from build123d import *

# Parameters (mm, degrees)
SKETCH1_W           = 250
SKETCH1_H           = 250
SKETCH1_R           = 1.5
BOSS_EXTRUDE1_DEPTH = 1.5
SKETCH2_R           = 2.25
SKETCH2_R_2         = 1.5
CUT_EXTRUDE1_DEPTH  = 2
CUT_EXTRUDE2_DEPTH  = 2
CUT_EXTRUDE3_DEPTH  = 2


with BuildPart() as part:
    # Sketch1 → Boss-Extrude1 (new body)
    with BuildSketch(Plane(origin=(0, 0, 0), x_dir=(1, 0, 0), z_dir=(0, 1, 0))):
        with Locations((-125, -125)):
            Rectangle(SKETCH1_W, SKETCH1_H)
        with Locations(Location((-125, -5.475, 0), (0, 0, 270))):
            Circle(SKETCH1_R, mode=Mode.SUBTRACT)
        with Locations(Location((-11.32496989, -88.064743747, 0), (0, 0, 270))):
            Circle(SKETCH1_R, mode=Mode.SUBTRACT)
        with Locations(Location((-54.74496772, -28.302243747, 0), (0, 0, 270))):
            Circle(SKETCH1_R, mode=Mode.SUBTRACT)
        with Locations(Location((-11.32496989, -161.935256253, 0), (0, 0, 270))):
            Circle(SKETCH1_R, mode=Mode.SUBTRACT)
        with Locations(Location((-54.74496772, -221.697756253, 0), (0, 0, 269.999999999))):
            Circle(SKETCH1_R, mode=Mode.SUBTRACT)
        with Locations(Location((-125, -244.525, 0), (0, 0, 270))):
            Circle(SKETCH1_R, mode=Mode.SUBTRACT)
        with Locations(Location((-195.25503228, -221.697756253, 0), (0, 0, 269.999999999))):
            Circle(SKETCH1_R, mode=Mode.SUBTRACT)
        with Locations(Location((-238.67503011, -161.935256253, 0), (0, 0, 270))):
            Circle(SKETCH1_R, mode=Mode.SUBTRACT)
        with Locations(Location((-238.67503011, -88.064743747, 0), (0, 0, 270))):
            Circle(SKETCH1_R, mode=Mode.SUBTRACT)
        with Locations(Location((-195.25503228, -28.302243747, 0), (0, 0, 270))):
            Circle(SKETCH1_R, mode=Mode.SUBTRACT)
    extrude(amount=BOSS_EXTRUDE1_DEPTH)

    # Sketch2 → Cut-Extrude1 (cut)
    with BuildSketch(Plane(origin=(0, 1.5, 0), x_dir=(1, 0, 0), z_dir=(0, 1, 0))):
        with Locations(Location((-212.5, -125, 0), (0, 0, 270))):
            Circle(SKETCH2_R)
        with Locations(Location((-228, -140.5, 0), (0, 0, 270))):
            Circle(SKETCH2_R_2)
        with Locations(Location((-228, -109.5, 0), (0, 0, 270))):
            Circle(SKETCH2_R_2)
        with Locations(Location((-197, -109.5, 0), (0, 0, 270))):
            Circle(SKETCH2_R_2)
        with Locations(Location((-197, -140.5, 0), (0, 0, 270))):
            Circle(SKETCH2_R_2)
    extrude(amount=-CUT_EXTRUDE1_DEPTH, mode=Mode.SUBTRACT)

    # Sketch3 → Cut-Extrude2 (cut)
    with BuildSketch(Plane(origin=(0, 1.5, 0), x_dir=(1, 0, 0), z_dir=(0, 1, 0))):
        with BuildLine():
            ThreePointArc((-245, -90), (-213.388347648, -36.611652352), (-160, -5))
            Line((-160, -5), (-245, -5))
            Line((-245, -5), (-245, -90))
        make_face()
        with BuildLine():
            ThreePointArc((-160, -245), (-213.388347648, -213.388347648), (-245, -160))
            Line((-245, -160), (-245, -245))
            Line((-245, -245), (-160, -245))
        make_face()
        with BuildLine():
            Line((-5, -245), (-5, -160))
            ThreePointArc((-5, -160), (-36.611652352, -213.388347648), (-90, -245))
            Line((-90, -245), (-5, -245))
        make_face()
        with BuildLine():
            Line((-5, -5), (-90, -5))
            ThreePointArc((-90, -5), (-36.611652352, -36.611652352), (-5, -90))
            Line((-5, -90), (-5, -5))
        make_face()
        with BuildLine():
            ThreePointArc((-10.95, -125), (-44.354471606, -44.354471606), (-125, -10.95))
            ThreePointArc((-125, -10.95), (-198.233880479, -37.568877109), (-237.282690117, -105))
            Line((-237.282690117, -105), (-232.5, -105))
            Line((-232.5, -105), (-192.5, -105))
            Line((-192.5, -105), (-192.5, -145))
            Line((-192.5, -145), (-232.5, -145))
            Line((-232.5, -145), (-237.282690117, -145))
            ThreePointArc((-237.282690117, -145), (-114.961033616, -238.607313382), (-10.95, -125))
        make_face()
    extrude(amount=-CUT_EXTRUDE2_DEPTH, mode=Mode.SUBTRACT)

    # Sketch4 → Cut-Extrude3 (cut)
    with BuildSketch(Plane(origin=(0, 1.5, 0), x_dir=(1, 0, 0), z_dir=(0, 1, 0))):
        with BuildLine():
            Line((-125, 0), (0, 0))
            Line((0, 0), (0, -125))
            ThreePointArc((0, -125), (-36.611652352, -36.611652352), (-125, 0))
        make_face()
    extrude(amount=-CUT_EXTRUDE3_DEPTH, mode=Mode.SUBTRACT)


solid = part.part
Can you work these out from the model? Positions are in its coordinate system, mm. Give positions to 0.01 mm unless a question says otherwise; leave off trailing zeros. Loops run counter-clockwise (first coordinate to the right, second up) from the corner with the lowest first, then second, coordinate; pieces in that order, holes last. Notation, with made-up numbers: (-6.5, 18) -> (13.5, 18) arc R24 cw to (13.5, 51) -> close; hole circle Ø9 at (60, 71.25). An arc over 180 degrees is marked (long way). Use one line per item in the form item = value.
1) We'd pull the mould along Z, two halves only. Please class faces 1 (the face through (-212.765, 0.76, 214.007)), 2 (the face through (-200, 1.5, 124)): released by +Z, released by -Z, zero draft, split by the parting line, or undercut.
Answers:
face_1 = undercut
face_2 = zero draft
2) If we section it at B-B (x = -33): Please give me the cut outline in (y, z).
Answers:
outline = (0, 40.38) -> (1.5, 40.38) -> (1.5, 57.6) -> (0, 57.6) -> close; (0, 192.4) -> (1.5, 192.4) -> (1.5, 209.62) -> (0, 209.62) -> close; (0, 245) -> (1.5, 245) -> (1.5, 250) -> (0, 250) -> close
3) Will this pin go through, and if not, where does the flat tip stop? pin 1 (2.5 mm diameter, centred on x = -228, z = 109.5, fed in from +Y) (3 decimals).
Answers:
pin_1 = through
4) I need wall thicknesses on line 1 along X through (y, z) = (0.6, 125); line 2 along X through (y, z) = (0.8, 76); line 3 along Z through (x, y) = (-43.5, 0.4). Which ranges of each line are inside material? Lowest first, please.
Answers:
line_1 = -250 to -214.75, -210.25 to -192.5, -10.95 to 0
line_2 = -250 to -245, -240 to -227.99, -22.01 to -10
line_3 = 30.22 to 45.22, 204.78 to 219.78, 245 to 250
5) If we section it at A-A (x = -163): Please give me the cut outline in (y, z), plus the area to 3 significant figures.
Answers:
outline = (0, 0) -> (1.5, 0) -> (1.5, 5) -> (0, 5) -> close; (0, 5.92) -> (1.5, 5.92) -> (1.5, 17.47) -> (0, 17.47) -> close; (0, 232.53) -> (1.5, 232.53) -> (1.5, 244.08) -> (0, 244.08) -> close; (0, 245) -> (1.5, 245) -> (1.5, 250) -> (0, 250) -> close
area = 49.7 mm²
6) If we section it at C-C (y = 1.1): Count the separate pieces of the cut face and the enclosed holes in it, plus the area to 3 significant figures.
Answers:
separate_pieces = 1
enclosed_holes = 19
area = 12,900 mm²
